```python
from build123d import *

# Parameters (mm, degrees)
SKETCH3_W           = 160
SKETCH3_H           = 80
BOSS_EXTRUDE1_DEPTH = 100
SKETCH5_R           = 12.5
CUT_EXTRUDE2_DEPTH  = 50


with BuildPart() as part:
    # Sketch1 → Revolve1 (revolve)
    with BuildSketch(Plane.XY):
        Polygon((0, 0), (-150, 0), (-150, 12), (-100, 12), (-100, 80), (0, 80), align=None)
    revolve(axis=Axis((0, 0, 0), (-1, 0, 0)))

    # Sketch3 → Boss-Extrude1 (add)
    with BuildSketch(Plane(origin=(0, 0, 0), x_dir=(0, 0, -1), z_dir=(1, 0, 0))):
        with Locations((0, -40)):
            Rectangle(SKETCH3_W, SKETCH3_H)
    extrude(amount=-BOSS_EXTRUDE1_DEPTH)

    # Sketch5 → Cut-Extrude2 (cut)
    with BuildSketch(Plane.XZ.offset(80)):
        with Locations((-50, 54.694760198)):
            Circle(SKETCH5_R)
        with Locations((-50, -65.305239802)):
            Circle(SKETCH5_R)
    extrude(amount=-CUT_EXTRUDE2_DEPTH, mode=Mode.SUBTRACT)


solid = part.part
```
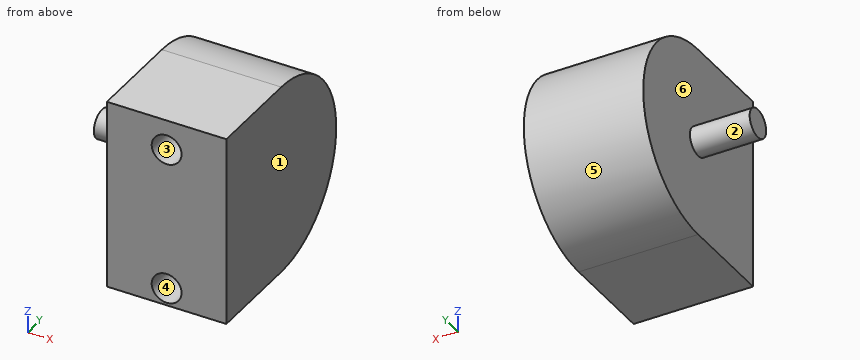
Geometry check sheet. Reference: the model listing, model coordinates, mm. Face numbers are marked on the shaded views. A direction names the side the tool comes from. Coordinates: 2 decimals unless noted, no trailing zeros. Order: outer loops, then holes, each group sorted by start corner. A loop starts at its lowest first (then second) coordinate and runs counter-clockwise, first axis right, second up. Notation, with made-up numbers: (81.5, 33.5) - (100.5, 33.5) arc R20 ccw to (100.5, 71.5) - close; hole circle Ø6 at (11.25, 3). An arc over 180 degrees is marked (long way). Answer as a JSON object with one key per item and string values. Group by question number.
Item 1: Sectioned sample at A-A, the plane z = 0. Record the cut outline in (x, y).
Item 2: Sectioned sample at D-D, the plane x = -35. Record the cut outline in (y, z).
Item 3: Tool access check on the marked faces 1 and 2. Record the directions out of +Z, -Z, +X, -X, +Y, -Y that give a thin tool (end or side, any length) a straight path to the whole face; none if there is none.
Item 4: Sectioned sample at B-B, the plane x = -50. Record the cut outline in (y, z).
Item 5: Depth check by flat-ended pin: pin 1 Ø1 at (x, y) = (-20.5, 36.5) entering from +Z; pin 2 Ø12.5 at (x, z) = (-51.5, 60.5) entering from -Y; pin 3 Ø6 at (y, z) = (-35, -9) entering from -X. Enter the tip coordinate at first touch or a pass-through.
Item 6: Sectioned sample at C-C, the plane y = -18. Record the cut outline in (x, z), and give its area (3 significant figures).
Item 7: Draft check along Z on the marked faces 3, 4, 5 and 6. Enter one of: +Z half, -Z half, draft (parallel to the pull), parting line (faces both ways), or undercut.
Item 8: Scan lines: probe 1 along Z at (x, y) = (-50, -46); probe 2 along X at (y, z) = (-59, 17); probe 3 along X at (y, z) = (-60.5, -57.5). Record each from-to range of solid material in increasing order.
Resolved:
{
 "1": {"outline": "(-150, -12) - (-100, -12) - (-100, -80) - (0, -80) - (0, 80) - (-100, 80) - (-100, 12) - (-150, 12) - close"},
 "2": {"outline": "(-80, -80) - (0, -80) arc R80 ccw to (0, 80) - (-80, 80) - close"},
 "3": {"face 1": "+Z, -Z, +X, +Y, -Y", "face 2": "-X"},
 "4": {"outline": "(-80, -80) - (0, -80) arc R80 ccw to (0, 80) - (-80, 80) - (-80, 67.19) - (-30, 67.19) - (-30, 42.19) - (-80, 42.19) - (-80, -52.81) - (-30, -52.81) - (-30, -77.81) - (-80, -77.81) - close"},
 "5": {"pin 1": "z = 71.44", "pin 2": "y = -30", "pin 3": "x = -100"},
 "6": {"outline": "(-100, -80) - (0, -80) - (0, 80) - (-100, 80) - close", "area": "16,000 mm^2"},
 "7": {"face 3": "undercut", "face 4": "undercut", "face 5": "parting line", "face 6": "draft"},
 "8": {"probe 1": "-80 to -77.81, -52.81 to 42.19, 67.19 to 80", "probe 2": "-100 to 0", "probe 3": "-100 to -59.76, -40.24 to 0"}
}
